Could you check a few things on this model? Use its own coordinates, in mm. A direction names the side the tool comes from. Give positions to 0.01 mm unless a question says otherwise; leave off trailing zeros. Loops run counter-clockwise (first coordinate to the right, second up) from the corner with the lowest first, then second, coordinate; pieces in that order, holes last. Notation, with made-up numbers: M 47,-13 L 99,-13 A24 ccw 99,14 Z; hole C 28,-2.75 d9. An arc over 180 degrees is marked long. Use a Markdown table: item, result. Add a question column.
1) If I drill on line 1 along X through (y, z) = (206, 2); line 2 along X through (y, z) = (1.5, 9); line 3 along Y through (x, z) = (-26.5, 0), over which ranges is the centre line in solid material (lowest first)? Write a range as [from, to].
2) Suppose I cut it at D-D on y = 105. List the corners of the cut face in (x, z) for me, and give its area (3 significant figures).
3) Suppose I cut it at C-C on z = 11. Count the separate pieces of the cut face and the enclosed holes in it, and give its area (3 significant figures).
4) Suppose I cut it at B-B on x = -53.5. List the corners of the cut face in (y, z) for me, and give its area (3 significant figures).
5) Suppose I cut it at A-A on z = -25.5. List the corners of the cut face in (x, y) for me.
6) We'd pull the mould along X, two halves only. Please class faces 1 (the flat face through (-67, 21, -10)), 2 (the flat face through (-16.383, 205, 0)), 3 (the flat face through (-43.811, 205, 0)): +X half, -X half, draft (parallel to the pull), parting line (faces both ways), or undercut.
7) Will these pins go through, and if not, where does the flat tip stop? pin 1 Ø5.5 at (x, y) = (-50.5, 43.5) entering from +Z; pin 2 Ø10 at (x, z) = (-47.5, -21.5) entering from -Y; pin 3 Ø20 at (x, z) = (-65.5, -9.5) entering from +Y; pin 4 Ø3 at (x, z) = (-55.5, -2) entering from -Y.
8) Which directions (+Z, -Z, +X, -X, +Y, -Y) give clear straight access to the entire face, cutting with the end or side of a thin tool? Please do faces 4 (the flat face through (-29, 210.307, 0)), 5 (the cylindrical face through (-0.867, 7.465, -3.905)), 6 (the cylindrical face through (-77.27, 44.54, -12.82)).
```python
from build123d import *

# Parameters (mm, degrees)
BOSS_EXTRUDE1_DEPTH = 17.5
SKETCH6_W           = 24.942027916
SKETCH6_H           = 10
SKETCH6_W_2         = 47.258134024
SKETCH6_H_2         = 15
CUT_EXTRUDE1_DEPTH  = 228.033901494
SKETCH7_R           = 25
CUT_EXTRUDE2_DEPTH  = 228.033901494
SKETCH8_R           = 4
CUT_EXTRUDE3_DEPTH  = 30
SKETCH10_R          = 4
CUT_EXTRUDE4_DEPTH  = 30
SKETCH11_W          = 7.160304618
SKETCH11_H          = 39.552070702
SKETCH11_H_2        = 22.637315958
BOSS_EXTRUDE2_DEPTH = 50
SKETCH13_R          = 4
CUT_EXTRUDE5_DEPTH  = 50
CUT_EXTRUDE6_DEPTH  = 50
CUT_EXTRUDE7_DEPTH  = 50
BOSS_EXTRUDE3_DEPTH = 70
SKETCH19_R          = 4
CUT_EXTRUDE8_DEPTH  = 70
SKETCH20_W          = 48.774167315
SKETCH20_H          = 27.556784468
CUT_EXTRUDE9_DEPTH  = 70
CUT_EXTRUDE10_DEPTH = 70
FILLET1_R           = 5
FILLET2_R           = 5
FILLET3_R           = 5
FILLET4_R           = 5


with BuildPart() as part:
    # Sketch1 → Boss-Extrude1 (new, symmetric)
    with BuildSketch(Plane.XY):
        Polygon((30, -10), (-30, -10), (-30, 140), (-43.810871114, 190), (-43.810871114, 220), (-13.810871114, 220), (-13.810871114, 190), (30, 140), align=None)
    extrude(amount=BOSS_EXTRUDE1_DEPTH, both=True)

    # Sketch6 → Cut-Extrude1 (cut, through all)
    with BuildSketch(Plane(origin=(0, 0, -17.5), x_dir=(-1, 0, 0), z_dir=(0, 0, -1))):
        with Locations((28.85405418, 190.307263481)):
            Rectangle(SKETCH6_W, SKETCH6_H)
        Rectangle(SKETCH6_W_2, SKETCH6_H)
        with Locations((0, 17.5)):
            Rectangle(SKETCH6_W_2, SKETCH6_H_2)
        with Locations((28.85405418, 205.307263481)):
            Rectangle(SKETCH6_W, SKETCH6_H)
    extrude(amount=-CUT_EXTRUDE1_DEPTH, mode=Mode.SUBTRACT)

    # Sketch7 → Cut-Extrude2 (cut, through all)
    with BuildSketch(Plane(origin=(0, 0, -17.5), x_dir=(-1, 0, 0), z_dir=(0, 0, -1))):
        with Locations((0, 105)):
            Circle(SKETCH7_R)
    extrude(amount=-CUT_EXTRUDE2_DEPTH, mode=Mode.SUBTRACT)

    # Sketch8 → Cut-Extrude3 (cut)
    with BuildSketch(Plane(origin=(0, 220, 0), x_dir=(1, 0, 0), z_dir=(0, 1, 0))):
        with Locations(Location((-28.860081831, 7.158757746, 0), (0, 0, 270))):
            Circle(SKETCH8_R)
    extrude(amount=-CUT_EXTRUDE3_DEPTH, mode=Mode.SUBTRACT)

    # Sketch10 → Cut-Extrude4 (cut)
    with BuildSketch(Plane.XZ.offset(10)):
        Circle(SKETCH10_R)
    extrude(amount=-CUT_EXTRUDE4_DEPTH, mode=Mode.SUBTRACT)

    # Sketch11 → Boss-Extrude2 (add)
    with BuildSketch(Plane(origin=(30, 0, 0), x_dir=(0, 0, -1), z_dir=(1, 0, 0))):
        with Locations((-0.000773436, 90.343921661)):
            Rectangle(SKETCH11_W, SKETCH11_H)
        with Locations((-0.000773436, 32.969473472)):
            Rectangle(SKETCH11_W, SKETCH11_H_2)
    extrude(amount=BOSS_EXTRUDE2_DEPTH)

    # Sketch13 → Cut-Extrude5 (cut)
    with BuildSketch(Plane.XY.offset(3.580925745)):
        with Locations((69.802457577, 90.343921661)):
            Circle(SKETCH13_R)
        with Locations((42.591748381, 32.969473472)):
            Circle(SKETCH13_R)
    extrude(amount=-CUT_EXTRUDE5_DEPTH, mode=Mode.SUBTRACT)

    # Sketch14 → Cut-Extrude6 (cut)
    with BuildSketch(Plane.XY.offset(3.580925745)):
        with BuildLine():
            Line((30, 110.119957012), (71.857382865, 97.843921661))
            ThreePointArc((71.857382865, 97.843921661), (77.47366635, 90.343921661), (71.857382865, 82.843921661))
            Line((71.857382865, 82.843921661), (30, 70.56788631))
            Line((30, 70.56788631), (80, 70.56788631))
            Line((80, 70.56788631), (80, 110.119957012))
            Line((80, 110.119957012), (30, 110.119957012))
        make_face()
    extrude(amount=-CUT_EXTRUDE6_DEPTH, mode=Mode.SUBTRACT)

    # Sketch15 → Cut-Extrude7 (cut)
    with BuildSketch(Plane.XY.offset(3.580925745)):
        with BuildLine():
            Line((30, 44.288131451), (43.349487429, 39.469473472))
            ThreePointArc((43.349487429, 39.469473472), (47.913726584, 32.969473472), (43.349487429, 26.469473472))
            Line((43.349487429, 26.469473472), (30, 21.650815493))
            Line((30, 21.650815493), (80, 21.650815493))
            Line((80, 21.650815493), (80, 44.288131451))
            Line((80, 44.288131451), (30, 44.288131451))
        make_face()
    extrude(amount=-CUT_EXTRUDE7_DEPTH, mode=Mode.SUBTRACT)

    # Sketch18 → Boss-Extrude3 (add)
    with BuildSketch(Plane.ZY.offset(30)):
        Polygon((11.672732765, 47), (-11.672732765, 47), (-38.952313989, 47), (-38.952313989, 42), (-11.672732765, 42), (11.672732765, 42), align=None)
        Polygon((-11.672732765, 26), (-38.952313989, 26), (-38.952313989, 21), (-11.672732765, 21), (11.672732765, 21), (11.672732765, 26), align=None)
    extrude(amount=BOSS_EXTRUDE3_DEPTH)

    # Sketch19 → Cut-Extrude8 (cut)
    with BuildSketch(Plane(origin=(0, 47, 0), x_dir=(1, 0, 0), z_dir=(0, 1, 0))):
        with Locations(Location((-85, 33, 0), (0, 0, 270))):
            Circle(SKETCH19_R)
    extrude(amount=-CUT_EXTRUDE8_DEPTH, mode=Mode.SUBTRACT)

    # Sketch20 → Cut-Extrude9 (cut)
    with BuildSketch(Plane.XZ.offset(-21)):
        with Locations((-54.387083657, -25.173921755)):
            Rectangle(SKETCH20_W, SKETCH20_H)
    extrude(amount=-CUT_EXTRUDE9_DEPTH, mode=Mode.SUBTRACT)

    # Sketch22 → Cut-Extrude10 (cut)
    with BuildSketch(Plane.XZ.offset(-21)):
        Polygon((-91.205371371, -38.952313989), (-91.205371371, 1.034470479), (-30, 1.034470479), (-30, 11.672732765), (-100, 11.672732765), (-100, -38.952313989), align=None)
    extrude(amount=-CUT_EXTRUDE10_DEPTH, mode=Mode.SUBTRACT)

    # Fillet1
    fillet1_edges = [part.edges().sort_by_distance(p)[0] for p in [
        (-78.774167315, 44.5, -11.395529521),
    ]]
    fillet(fillet1_edges, radius=FILLET1_R)

    # Fillet2
    fillet2_edges = [part.edges().sort_by_distance(p)[0] for p in [
        (-78.774167315, 23.5, -11.395529521),
    ]]
    fillet(fillet2_edges, radius=FILLET2_R)

    # Fillet3
    fillet3_edges = [part.edges().sort_by_distance(p)[0] for p in [
        (-91.205371371, 44.5, 1.034470479),
        (-91.205371371, 23.5, 1.034470479),
    ]]
    fillet(fillet3_edges, radius=FILLET3_R)

    # Fillet4
    fillet4_edges = [part.edges().sort_by_distance(p)[0] for p in [
        (-41.325068138, 185.307263481, 0),
        (-16.383040222, 185.307263481, 0),
        (-16.383040222, 195.307263481, 0),
        (-41.325068138, 195.307263481, 0),
    ]]
    fillet(fillet4_edges, radius=FILLET4_R - 0.0001)  # a hair under: the kernel refuses the full size


solid = part.part
```
Answer block:
| question | item | result |
|---|---|---|
| 1 | line 1 | x = [-43.81, -41.33], [-16.38, -13.81] |
| 1 | line 2 | x = [-30, -23.63], [23.63, 30] |
| 1 | line 3 | y = [-10, 185.31], [195.31, 200.31], [210.31, 220] |
| 2 | outline | M -30,-17.5 L -25,-17.5 L -25,17.5 L -30,17.5 Z; M 25,-17.5 L 30,-17.5 L 30,-3.58 L 47.46,-3.58 L 47.46,3.58 L 30,3.58 L 30,17.5 L 25,17.5 Z |
| 2 | area | 475 mm^2 |
| 3 | separate pieces | 1 |
| 3 | enclosed holes | 5 |
| 3 | area | 8,530 mm^2 |
| 4 | outline | M 21,-11.4 L 26,-11.4 L 26,1.03 L 21,1.03 Z; M 42,-11.4 L 47,-11.4 L 47,1.03 L 42,1.03 Z |
| 4 | area | 124 mm^2 |
| 5 | outline | M -91.21,21 L -78.77,21 L -78.77,26 L -91.21,26 Z; M -91.21,42 L -78.77,42 L -78.77,47 L -91.21,47 Z |
| 6 | face 1 | draft |
| 6 | face 2 | undercut |
| 6 | face 3 | -X half |
| 7 | pin 1 | stops at z = 1.03 |
| 7 | pin 2 | passes through |
| 7 | pin 3 | stops at y = 47 |
| 7 | pin 4 | stops at y = 21 |
| 8 | face 4 | +Z, -Z |
| 8 | face 5 | -Y |
| 8 | face 6 | -Z, +Y, -Y |
